from build123d import *

# Parameters (mm, degrees)
SKETCH1_W           = 1219.2
SKETCH1_H           = 635
BOSS_EXTRUDE2_DEPTH = 330.2
SKETCH3_W           = 1219.2
SKETCH3_H           = 101.6
CUT_EXTRUDE1_DEPTH  = 596.9
FILLET2_R           = 17.78
CUT_EXTRUDE2_DEPTH  = 226.06
FILLET4_R           = 44.45
CUT_EXTRUDE3_DEPTH  = 1.27
FILLET5_R           = 12.7
CUT_EXTRUDE4_DEPTH  = 608.33
CUT_EXTRUDE6_DEPTH  = 316.23
SKETCH12_W          = 635
SKETCH12_H          = 190.5
CUT_EXTRUDE7_DEPTH  = 2.54
SKETCH13_W          = 635
SKETCH13_H          = 190.5
CUT_EXTRUDE8_DEPTH  = 2.54
SKETCH15_R          = 25.4
CUT_EXTRUDE9_DEPTH  = 6.35
CUT_EXTRUDE10_START = -1219.2
CUT_EXTRUDE10_DEPTH = 1219.2


with BuildPart() as part:
    # Sketch1 → Boss-Extrude2 (new body)
    with BuildSketch(Plane(origin=(0, 0, 0), x_dir=(1, 0, 0), z_dir=(0, 1, 0))):
        Rectangle(SKETCH1_W, SKETCH1_H)
    extrude(amount=BOSS_EXTRUDE2_DEPTH)

    # Sketch3 → Cut-Extrude1 (cut)
    with BuildSketch(Plane.XY.offset(317.5)):
        with Locations((0, 279.4)):
            Rectangle(SKETCH3_W, SKETCH3_H)
    extrude(amount=-CUT_EXTRUDE1_DEPTH, mode=Mode.SUBTRACT)

    # Fillet2
    fillet2_edges = [part.edges().sort_by_distance(p)[0] for p in [
        (0, 228.6, -279.4),
    ]]
    fillet(fillet2_edges, radius=FILLET2_R)

    # Sketch5 → Cut-Extrude2 (cut)
    with BuildSketch(Plane(origin=(0, 228.6, 0), x_dir=(1, 0, 0), z_dir=(0, 1, 0))):
        with BuildLine():
            Line((95.25, 152.4), (488.95, 152.4))
            ThreePointArc((488.95, 152.4), (520.380896424, 139.380896424), (533.4, 107.95))
            Line((533.4, 107.95), (533.4, -209.55))
            ThreePointArc((533.4, -209.55), (520.380896424, -240.980896424), (488.95, -254))
            Line((488.95, -254), (95.25, -254))
            ThreePointArc((95.25, -254), (63.819103576, -240.980896424), (50.8, -209.55))
            Line((50.8, -209.55), (50.8, 107.95))
            ThreePointArc((50.8, 107.95), (63.819103576, 139.380896424), (95.25, 152.4))
        make_face()
    extrude(amount=-CUT_EXTRUDE2_DEPTH, mode=Mode.SUBTRACT)

    # Fillet4
    fillet4_edges = [part.edges().sort_by_distance(p)[0] for p in [
        (520.380896424, 2.54, -139.380896424),
        (533.4, 2.54, 50.8),
        (520.380896424, 2.54, 240.980896424),
        (292.1, 2.54, 254),
        (63.819103576, 2.54, 240.980896424),
        (50.8, 2.54, 50.8),
        (63.819103576, 2.54, -139.380896424),
        (292.1, 2.54, -152.4),
    ]]
    fillet(fillet4_edges, radius=FILLET4_R)

    # Sketch7 → Cut-Extrude3 (cut)
    with BuildSketch(Plane(origin=(0, 228.6, 0), x_dir=(1, 0, 0), z_dir=(0, 1, 0))):
        with BuildLine():
            Line((-571.5, -292.1), (571.5, -292.1))
            ThreePointArc((571.5, -292.1), (580.480256121, -288.380256121), (584.2, -279.4))
            Line((584.2, -279.4), (584.2, 223.52))
            ThreePointArc((584.2, 223.52), (580.480256121, 232.500256121), (571.5, 236.22))
            Line((571.5, 236.22), (-571.5, 236.22))
            ThreePointArc((-571.5, 236.22), (-580.480256121, 232.500256121), (-584.2, 223.52))
            Line((-584.2, 223.52), (-584.2, -279.4))
            ThreePointArc((-584.2, -279.4), (-580.480256121, -288.380256121), (-571.5, -292.1))
        make_face()
    extrude(amount=-CUT_EXTRUDE3_DEPTH, mode=Mode.SUBTRACT)

    # Fillet5
    # the kernel refuses this fillet: 12.7 mm, written as the material it adds along each edge
    with BuildSketch(Plane(origin=(-571.5, 227.33, 292.1), x_dir=(0, 0, -1), z_dir=(1, 0, 0)), Plane(origin=(571.5, 227.33, -236.22), x_dir=(0, 0, 1), z_dir=(-1, 0, 0))) as fillet5_piece_1:
        with BuildLine():
            CenterArc((5.535801658, 12.7), FILLET5_R, 244.158067237, 25.841932763)
            Line((0, 1.27), (0, 0))
            Line((0, 0), (5.535801658, 0))
        make_face()
    extrude(amount=1143)
    with BuildSketch(Plane(origin=(-571.5, 227.33, 279.4), x_dir=(-1, 0, 0), z_dir=(0, 0, -1))) as fillet5_piece_2:
        with BuildLine():
            CenterArc((7.164198342, 12.7), FILLET5_R, 270, 25.841932763)
            Line((12.7, 1.27), (12.7, 0))
            Line((12.7, 0), (7.164198342, 0))
        make_face()
    revolve(axis=Axis((-571.5, 227.33, 279.4), (0, 1, 0)), revolution_arc=90)
    with BuildSketch(Plane(origin=(-584.2, 227.33, -223.52), x_dir=(1, 0, 0), z_dir=(0, 0, 1)), Plane(origin=(584.2, 227.33, 279.4), x_dir=(-1, 0, 0), z_dir=(0, 0, -1))) as fillet5_piece_3:
        with BuildLine():
            CenterArc((5.535801658, 12.7), FILLET5_R, 244.158067237, 25.841932763)
            Line((0, 1.27), (0, 0))
            Line((0, 0), (5.535801658, 0))
        make_face()
    extrude(amount=502.92)
    with BuildSketch(Plane(origin=(-571.5, 227.33, -223.52), x_dir=(0, 0, -1), z_dir=(1, 0, 0))) as fillet5_piece_4:
        with BuildLine():
            CenterArc((7.164198342, 12.7), FILLET5_R, 270, 25.841932763)
            Line((12.7, 1.27), (12.7, 0))
            Line((12.7, 0), (7.164198342, 0))
        make_face()
    revolve(axis=Axis((-571.5, 227.33, -223.52), (0, 1, 0)), revolution_arc=90)
    with BuildSketch(Plane(origin=(571.5, 227.33, -223.52), x_dir=(1, 0, 0), z_dir=(0, 0, 1))) as fillet5_piece_5:
        with BuildLine():
            CenterArc((7.164198342, 12.7), FILLET5_R, 270, 25.841932763)
            Line((12.7, 1.27), (12.7, 0))
            Line((12.7, 0), (7.164198342, 0))
        make_face()
    revolve(axis=Axis((571.5, 227.33, -223.52), (0, 1, 0)), revolution_arc=90)
    with BuildSketch(Plane(origin=(571.5, 227.33, 279.4), x_dir=(0, 0, 1), z_dir=(-1, 0, 0))) as fillet5_piece_6:
        with BuildLine():
            CenterArc((7.164198342, 12.7), FILLET5_R, 270, 25.841932763)
            Line((12.7, 1.27), (12.7, 0))
            Line((12.7, 0), (7.164198342, 0))
        make_face()
    revolve(axis=Axis((571.5, 227.33, 279.4), (0, 1, 0)), revolution_arc=90)
    # the kernel refuses this fillet: 12.7 mm, written as the material it takes off along each edge
    with BuildSketch(Plane(origin=(488.95, 227.33, -107.95), x_dir=(1, 0, 0), z_dir=(0, 0, 1))) as fillet5_2_piece_1:
        with BuildLine():
            CenterArc((44.45 + FILLET5_R, -FILLET5_R), FILLET5_R, 90, 90)
            Line((44.45, -FILLET5_R), (44.45, 0))
            Line((44.45, 0), (44.45 + FILLET5_R, 0))
        make_face()
    revolve(axis=Axis((488.95, 227.33, -107.95), (0, 1, 0)), revolution_arc=90, mode=Mode.SUBTRACT)
    with BuildSketch(Plane(origin=(488.95, 227.33, -152.4), x_dir=(0, 0, -1), z_dir=(-1, 0, 0)), Plane(origin=(95.25, 227.33, 254), x_dir=(0, 0, 1), z_dir=(1, 0, 0))) as fillet5_2_piece_2:
        with BuildLine():
            CenterArc((FILLET5_R, FILLET5_R), FILLET5_R, 180, 90)
            Line((0, FILLET5_R), (0, 0))
            Line((0, 0), (FILLET5_R, 0))
        make_face()
    extrude(amount=393.7, mode=Mode.SUBTRACT)
    with BuildSketch(Plane(origin=(95.25, 227.33, -107.95), x_dir=(0, 0, -1), z_dir=(1, 0, 0))) as fillet5_2_piece_3:
        with BuildLine():
            CenterArc((44.45 + FILLET5_R, -FILLET5_R), FILLET5_R, 90, 90)
            Line((44.45, -FILLET5_R), (44.45, 0))
            Line((44.45, 0), (44.45 + FILLET5_R, 0))
        make_face()
    revolve(axis=Axis((95.25, 227.33, -107.95), (0, 1, 0)), revolution_arc=90, mode=Mode.SUBTRACT)
    with BuildSketch(Plane(origin=(50.8, 227.33, -107.95), x_dir=(0, -1, 0), z_dir=(0, 0, 1))) as fillet5_2_piece_4:
        with BuildLine():
            CenterArc((FILLET5_R, -FILLET5_R), FILLET5_R, 90, 90)
            Line((0, -FILLET5_R), (0, 0))
            Line((0, 0), (FILLET5_R, 0))
        make_face()
    extrude(amount=317.5, mode=Mode.SUBTRACT)
    with BuildSketch(Plane(origin=(95.25, 227.33, 209.55), x_dir=(-1, 0, 0), z_dir=(0, 0, -1))) as fillet5_2_piece_5:
        with BuildLine():
            CenterArc((44.45 + FILLET5_R, -FILLET5_R), FILLET5_R, 90, 90)
            Line((44.45, -FILLET5_R), (44.45, 0))
            Line((44.45, 0), (44.45 + FILLET5_R, 0))
        make_face()
    revolve(axis=Axis((95.25, 227.33, 209.55), (0, 1, 0)), revolution_arc=90, mode=Mode.SUBTRACT)
    with BuildSketch(Plane(origin=(488.95, 227.33, 209.55), x_dir=(0, 0, 1), z_dir=(-1, 0, 0))) as fillet5_2_piece_6:
        with BuildLine():
            CenterArc((44.45 + FILLET5_R, -FILLET5_R), FILLET5_R, 90, 90)
            Line((44.45, -FILLET5_R), (44.45, 0))
            Line((44.45, 0), (44.45 + FILLET5_R, 0))
        make_face()
    revolve(axis=Axis((488.95, 227.33, 209.55), (0, 1, 0)), revolution_arc=90, mode=Mode.SUBTRACT)
    with BuildSketch(Plane(origin=(533.4, 227.33, 209.55), x_dir=(1, 0, 0), z_dir=(0, 0, -1))) as fillet5_2_piece_7:
        with BuildLine():
            CenterArc((FILLET5_R, FILLET5_R), FILLET5_R, 180, 90)
            Line((0, FILLET5_R), (0, 0))
            Line((0, 0), (FILLET5_R, 0))
        make_face()
    extrude(amount=317.5, mode=Mode.SUBTRACT)

    # Sketch9 → Cut-Extrude4 (cut, symmetric)
    with BuildSketch(Plane(origin=(0, 0, 0), x_dir=(0, 0, -1), z_dir=(1, 0, 0))):
        with BuildLine():
            Line((317.5, 226.06), (198.12, 226.06))
            ThreePointArc((198.12, 226.06), (166.689103576, 213.040896424), (153.67, 181.61))
            Line((153.67, 181.61), (153.67, 45.72))
            ThreePointArc((153.67, 45.72), (140.650896424, 14.289103576), (109.22, 1.27))
            Line((109.22, 1.27), (-210.82, 1.27))
            ThreePointArc((-210.82, 1.27), (-242.250896424, 14.289103576), (-255.27, 45.72))
            Line((-255.27, 45.72), (-255.27, 181.61))
            ThreePointArc((-255.27, 181.61), (-268.289103576, 213.040896424), (-299.72, 226.06))
            Line((-299.72, 226.06), (-316.23, 226.06))
            Line((-316.23, 226.06), (-316.23, 190.5))
            Line((-316.23, 190.5), (-317.5, 190.5))
            Line((-317.5, 190.5), (-317.5, 0))
            Line((-317.5, 0), (317.5, 0))
            Line((317.5, 0), (317.5, 226.06))
        make_face()
    extrude(amount=CUT_EXTRUDE4_DEPTH, both=True, mode=Mode.SUBTRACT)

    # Sketch11 → Cut-Extrude6 (cut, symmetric)
    with BuildSketch(Plane.XY):
        with BuildLine():
            Line((-608.33, 226.06), (5.08, 226.06))
            ThreePointArc((5.08, 226.06), (36.510896424, 213.040896424), (49.53, 181.61))
            Line((49.53, 181.61), (49.53, 45.72))
            ThreePointArc((49.53, 45.72), (62.549103576, 14.289103576), (93.98, 1.27))
            Line((93.98, 1.27), (-608.33, 1.27))
            Line((-608.33, 1.27), (-608.33, 226.06))
        make_face()
        with BuildLine():
            Line((534.67, 45.72), (534.67, 181.61))
            ThreePointArc((534.67, 181.61), (547.689103576, 213.040896424), (579.12, 226.06))
            Line((579.12, 226.06), (608.33, 226.06))
            Line((608.33, 226.06), (608.33, 1.27))
            Line((608.33, 1.27), (490.22, 1.27))
            ThreePointArc((490.22, 1.27), (521.650896424, 14.289103576), (534.67, 45.72))
        make_face()
    extrude(amount=CUT_EXTRUDE6_DEPTH, both=True, mode=Mode.SUBTRACT)

    # Sketch12 → Cut-Extrude7 (cut)
    with BuildSketch(Plane.ZY.offset(609.6)):
        with Locations((0, 95.25)):
            Rectangle(SKETCH12_W, SKETCH12_H)
    extrude(amount=-CUT_EXTRUDE7_DEPTH, mode=Mode.SUBTRACT)

    # Sketch13 → Cut-Extrude8 (cut)
    with BuildSketch(Plane(origin=(609.6, 0, 0), x_dir=(0, 0, -1), z_dir=(1, 0, 0))):
        with Locations((0, 95.25)):
            Rectangle(SKETCH13_W, SKETCH13_H)
    extrude(amount=-CUT_EXTRUDE8_DEPTH, mode=Mode.SUBTRACT)

    # Sketch16 → Revolve1 (revolve)
    with BuildSketch(Plane(origin=(292.1, 0, 0), x_dir=(0, 0, -1), z_dir=(1, 0, 0)), mode=Mode.PRIVATE) as revolve1_sk:
        with BuildLine():
            Line((38.1, 1.27), (38.1, -3.81))
            Line((38.1, -3.81), (77.47, -3.81))
            ThreePointArc((77.47, -3.81), (86.098103461, -0.38238846), (95.25, 1.178213968))
            Line((95.25, 1.178213968), (95.25, 1.27))
            Line((95.25, 1.27), (38.1, 1.27))
        make_face()
    revolve(revolve1_sk.sketch.rotate(Axis((292.1, 1.27, -38.1), (0, -1, 0)), 180), axis=Axis((292.1, 1.27, -38.1), (0, -1, 0)))

    # Sketch15 → Cut-Extrude9 (cut)
    with BuildSketch(Plane(origin=(0, 2.54, 0), x_dir=(1, 0, 0), z_dir=(0, 1, 0))):
        with Locations(Location((292.1, 38.1, 0), (0, 0, 270))):
            Circle(SKETCH15_R)
    extrude(amount=-CUT_EXTRUDE9_DEPTH, mode=Mode.SUBTRACT)

    # Sketch17 → Cut-Extrude10 (cut)
    with BuildSketch(Plane(origin=(609.6, 0, 0), x_dir=(0, 0, -1), z_dir=(1, 0, 0)).offset(CUT_EXTRUDE10_START)):
        Polygon((317.5, 292.1), (311.15, 266.7), (311.15, 215.9), (317.5, 190.5), align=None)
    extrude(amount=CUT_EXTRUDE10_DEPTH, mode=Mode.SUBTRACT)


solid = part.part
Could you check a few things on this model? Use its own coordinates, in mm. A direction names the side the tool comes from. Give positions to 0.01 mm unless a question says otherwise; leave off trailing zeros. Order: outer loops, then holes, each group sorted by start corner. A loop starts at its lowest first (then second) coordinate and runs counter-clockwise, first axis right, second up. Notation, with made-up numbers: (49.5, 10.5) - (72.5, 10.5) arc R25 ccw to (72.5, 25.5) - close; hole circle Ø4 at (10.5, 51). An arc over 180 degrees is marked (long way). One line per item, written item: value. Start each with the question number.
1. Imagine slicing it at A-A on z = 100. List the corners of the cut face in (x, y) for me.
2. Imagine slicing it at C-C on x = -228. List the corners of the cut face in (y, z) for me, plus the area to 3 significant figures.
3. For faces 1 (the face through (534.67, 113, 54)), 2 (the face through (64.167, 131.983, 241.325)), 3 (the face through (-9, 209, 317.5)), 4 (the face through (-608.33, 209, 4)), which set-ups out of +Z, -Z, +X, -X, +Y, -Y let a thin tool reach every point of the face, with its end or its side?
4. Thinking about a two-plate mould opening in Z: for faces 5 (the face through (296.118, 213.385, -167.037)), 6 (the face through (-9, 289, -279.4)), 7 (the face through (520.033, 131.983, -139.725)), 8 (the face through (609.6, 224, -46)), which applies, +Z half, -Z half, draft (parallel to the pull), parting line (faces both ways), or undercut?
5. If I drill on probe 1 along Y at (x, z) = (118.5, 85); probe 2 along Z at (x, y) = (-144.5, 301); probe 3 along Z at (x, y) = (379, 122.5), over which ranges is the centre line in solid material (lowest first)?
6. Imagine slicing it at B-B on y = 170. List the corners of the cut face in (x, z) for me.
7. For P1, Ø3, axis at y = 231.5, z = 168, coming from the +X side; P2, Ø8, axis at y = 122, z = 212.5, coming from the -X side; P3, Ø1, axis at x = -190, z = -214, coming from the -Y side; P4, Ø10, axis at x = 426.5, z = -116, coming from the -Y side, each with a flat end and sliding along its axis, tell me the tip position at first contact or that it passes through.
Values:
1. outline: (-609.6, 190.5) - (-608.33, 190.5) - (-608.33, 226.06) - (5.08, 226.06) arc R44.45 cw to (49.53, 181.61) - (49.53, 45.72) arc R44.45 ccw to (93.98, 1.27) - (490.22, 1.27) arc R44.45 ccw to (534.67, 45.72) - (534.67, 181.61) arc R44.45 cw to (579.12, 226.06) - (608.33, 226.06) - (608.33, 190.5) - (609.6, 190.5) - (609.6, 228.6) - (584.2, 228.6) arc R12.7 cw to (578.66, 227.33) - (546.1, 227.33) arc R12.7 ccw to (533.4, 214.63) - (533.4, 46.99) arc R44.45 cw to (488.95, 2.54) - (95.25, 2.54) arc R44.45 cw to (50.8, 46.99) - (50.8, 214.63) arc R12.7 ccw to (38.1, 227.33) - (-578.66, 227.33) arc R12.7 cw to (-584.2, 228.6) - (-609.6, 228.6) - close
2. outline: (190.5, 316.23) - (226.06, 316.23) - (226.06, -311.15) - (266.7, -311.15) - (292.1, -317.5) - (330.2, -317.5) - (330.2, -279.4) - (246.38, -279.4) arc R17.78 cw to (228.6, -261.62) - (228.6, -236.22) arc R12.7 cw to (227.33, -230.68) - (227.33, 286.56) arc R12.7 cw to (228.6, 292.1) - (228.6, 317.5) - (190.5, 317.5) - close
2. area: 4,590 mm²
3. face 1: +Z, -Z, +X, -Y
3. face 2: +Y
3. face 3: +Z, +X, -X, +Y, -Y
3. face 4: -Z, -Y
4. face 5: -Z half
4. face 6: +Z half
4. face 7: undercut
4. face 8: draft
5. probe 1: 1.27 to 2.54
5. probe 2: -317.5 to -279.4
5. probe 3: -153.67 to -152.4, 254 to 255.27
6. outline: (49.53, -153.67) - (534.67, -153.67) - (534.67, 255.27) - (49.53, 255.27) - close; hole (50.8, -107.95) arc R44.45 ccw to (95.25, -152.4) - (488.95, -152.4) arc R44.45 ccw to (533.4, -107.95) - (533.4, 209.55) arc R44.45 ccw to (488.95, 254) - (95.25, 254) arc R44.45 ccw to (50.8, 209.55) - close
7. P1: through
7. P2: x = 49.53
7. P3: y = 226.06
7. P4: y = 1.31
